Verification items for this drawing (mm, ordinates from the low corner). A direction names the side the tool comes from. Coordinates: 2 decimals unless noted, no trailing zeros. Order: outer loops, then holes, each group sorted by start corner. A loop starts at its lowest first (then second) coordinate and runs counter-clockwise, first axis right, second up.
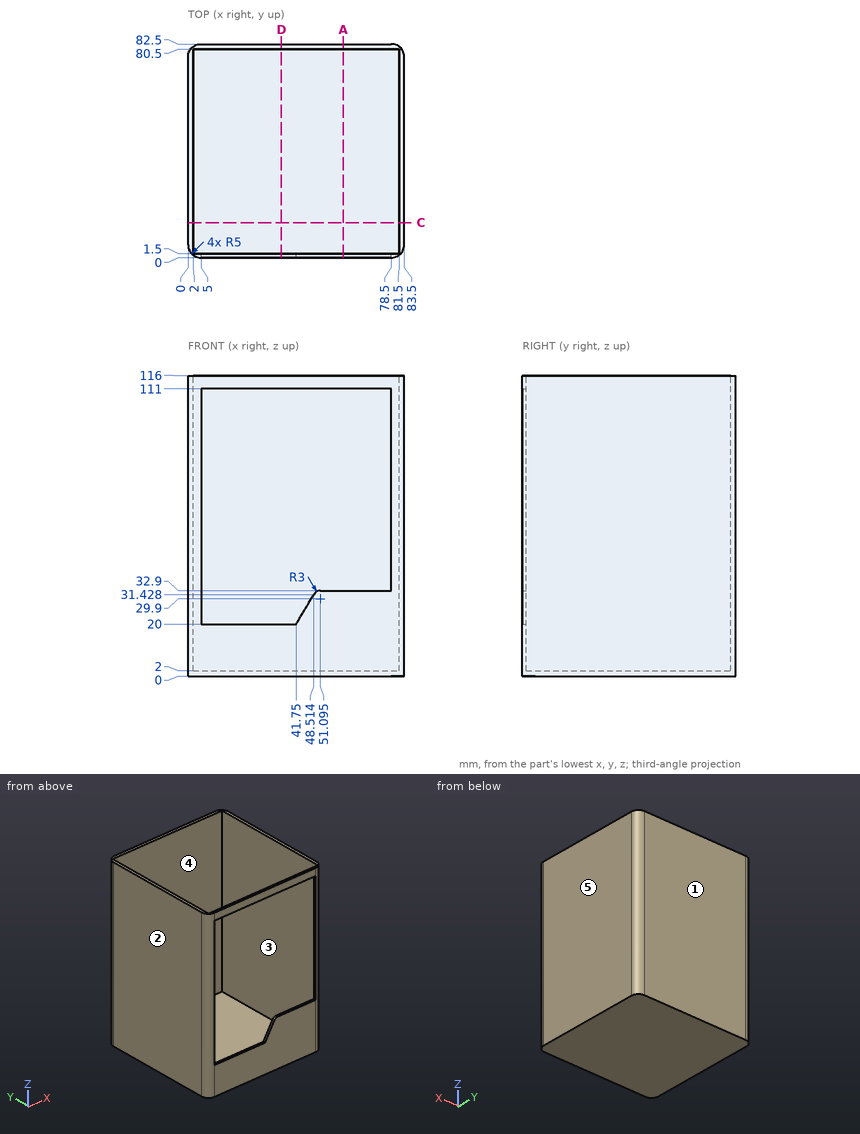
Item 1: Sectioned sample at A-A (x = 60). Record the cut outline in (y, z).
Item 2: Depth check by flat-ended pin: P1, Ø1.6, axis at y = 0.5, z = 53.5, coming from the +X side; P2, Ø1, axis at x = 51.5, z = 41.5, coming from the -Y side; P3, Ø1.5, axis at x = 9, y = 34, coming from the +Z side. Enter the tip coordinate at first touch or a pass-through.
Item 3: Tool access check on the marked faces 4 and 5. Record the directions out of +Z, -Z, +X, -X, +Y, -Y that give a thin tool (end or side, any length) a straight path to the whole face; none if there is none.
Item 4: Sectioned sample at D-D (x = 36). Record the cut outline in (y, z).
Item 5: Sectioned sample at C-C (y = 13.5). Record the cut outline in (x, z).
Item 6: Release check for a two-part mould opening along Y. For the marked faces 1, 2 and 3 record: pulls with the +Y half, pulls with the -Y half, needs draft (parallel to the pull), parting line crosses it, or undercut.
Item 7: Thickness scan on line 1 along X through (y, z) = (13.5, 86.5); line 2 along Y through (x, z) = (35, 12.5); line 3 along Y through (x, z) = (21, 110.5). Record the ranges inside material, lowest first.
Geometry check:
1. outline: (0, 0) - (82.5, 0) - (82.5, 116) - (80.5, 116) - (80.5, 2) - (1.5, 2) - (1.5, 32.9) - (0, 32.9) - close; (0, 111) - (1.5, 111) - (1.5, 116) - (0, 116) - close
2. P1: stops at x = 81.86
2. P2: stops at y = 80.5
2. P3: stops at z = 2
3. face 4: +Z
3. face 5: +Z, -Z, +X, +Y, -Y
4. outline: (0, 0) - (82.5, 0) - (82.5, 116) - (80.5, 116) - (80.5, 2) - (1.5, 2) - (1.5, 20) - (0, 20) - close; (0, 111) - (1.5, 111) - (1.5, 116) - (0, 116) - close
5. outline: (0, 0) - (83.5, 0) - (83.5, 116) - (81.5, 116) - (81.5, 2) - (2, 2) - (2, 116) - (0, 116) - close
6. face 1: pulls with the +Y half
6. face 2: needs draft
6. face 3: undercut
7. line 1: x = 0 to 2, 81.5 to 83.5
7. line 2: y = 0 to 1.5, 80.5 to 82.5
7. line 3: y = 80.5 to 82.5
